from build123d import *

# Parameters (mm, degrees)
SKETCH2_W                      = 127
SKETCH2_H                      = 76.2
BOSS_EXTRUDE2_DEPTH            = 76.2
FILLET1_R                      = 12.7
CHAMFER1_SIZE                  = 10
F_3_4_0_7500_DOWEL_HOLE1_D     = 19.05
F_3_4_0_7500_DOWEL_HOLE1_DEPTH = 76.2
F_3_4_0_7500_DOWEL_HOLE1_TIP   = 5.723197396
SKETCH9_W                      = 38.1
SKETCH9_H                      = 38.1
BOSS_EXTRUDE3_DEPTH            = 76.2
SKETCH10_R                     = 6.355
CUT_EXTRUDE1_DEPTH             = 175.711569487
FILLET3_R                      = 4.76


# Read off the part's stored shape, not the designer's step: 1/4-20 Tapped Hole1
with BuildPart() as part:
    # Sketch2 → Boss-Extrude2 (new body)
    with BuildSketch(Plane(origin=(0, 0, 0), x_dir=(1, 0, 0), z_dir=(0, 1, 0))):
        Rectangle(SKETCH2_W, SKETCH2_H)
    extrude(amount=BOSS_EXTRUDE2_DEPTH)

    # Fillet1
    fillet1_edges = [part.edges().sort_by_distance(p)[0] for p in [
        (-63.5, 76.2, 0),
        (-63.5, 0, 0),
    ]]
    fillet(fillet1_edges, radius=FILLET1_R)

    # Chamfer1
    chamfer1_edges = [part.edges().sort_by_distance(p)[0] for p in [
        (-63.5, 38.1, 38.1),
        (-63.5, 38.1, -38.1),
        (6.35, 0, 38.1),
        (6.35, 76.2, 38.1),
        (-59.780256121, 72.480256121, 38.1),
        (-59.780256121, 3.719743879, 38.1),
        (-59.780256121, 72.480256121, -38.1),
        (-59.780256121, 3.719743879, -38.1),
        (6.35, 0, -38.1),
        (6.35, 76.2, -38.1),
    ]]
    chamfer(chamfer1_edges, length=CHAMFER1_SIZE)

    # 3/4 (0.7500) Dowel Hole1
    with Locations(Plane(origin=(63.5, 0, 0), x_dir=(0, 0, -1), z_dir=(1, 0, 0))):
        with Locations((0, 36.890636669)):
            Hole(F_3_4_0_7500_DOWEL_HOLE1_D / 2, depth=F_3_4_0_7500_DOWEL_HOLE1_DEPTH)
            with Locations((0, 0, -(F_3_4_0_7500_DOWEL_HOLE1_DEPTH + F_3_4_0_7500_DOWEL_HOLE1_TIP / 2))):  # 118° drill point
                Cone(0, F_3_4_0_7500_DOWEL_HOLE1_D / 2, F_3_4_0_7500_DOWEL_HOLE1_TIP, mode=Mode.SUBTRACT)

    # 1/4-20 Tapped Hole1 outline → 1/4-20 Tapped Hole1 (revolve, cut)
    with BuildSketch(Plane(origin=(9.290251981, 0, 0), x_dir=(1, 0, 0), z_dir=(0, 0, 1))):
        Polygon((2.5527, 0), (2.5527, 27.365636669), (2.145213678, 27.610479152), (0, 27.610479152), (0, 0), align=None)
    revolve(axis=Axis((9.290251981, 0, 0), (0, 1, 0)), mode=Mode.SUBTRACT)

    # 1_4-20 Tapped Hole1 2 outline → 1_4-20 Tapped Hole1 2 (revolve, cut)
    with BuildSketch(Plane(origin=(36.474004082, 0, 0), x_dir=(1, 0, 0), z_dir=(0, 0, 1))):
        Polygon((2.5527, 0), (2.5527, 27.365636669), (2.145213678, 27.610479152), (0, 27.610479152), (0, 0), align=None)
    revolve(axis=Axis((36.474004082, 0, 0), (0, 1, 0)), mode=Mode.SUBTRACT)

    # Sketch9 → Boss-Extrude3 (add)
    with BuildSketch(Plane(origin=(0, 76.2, 0), x_dir=(1, 0, 0), z_dir=(0, 1, 0))):
        Rectangle(SKETCH9_W, SKETCH9_H)
    extrude(amount=BOSS_EXTRUDE3_DEPTH)

    # Sketch10 → Cut-Extrude1 (cut, through all)
    with BuildSketch(Plane.XY.offset(19.05)):
        with Locations((0, 98.552)):
            Circle(SKETCH10_R)
        with Locations((0, 130.302)):
            Circle(SKETCH10_R)
    extrude(amount=-CUT_EXTRUDE1_DEPTH, mode=Mode.SUBTRACT)

    # Fillet3
    fillet3_edges = [part.edges().sort_by_distance(p)[0] for p in [
        (19.05, 114.3, 19.05),
        (19.05, 114.3, -19.05),
        (-19.05, 114.3, -19.05),
        (-19.05, 114.3, 19.05),
    ]]
    fillet(fillet3_edges, radius=FILLET3_R)


solid = part.part
Input: part model. Units: mm. Frame: model coordinates. A direction names the side the tool comes from. Coordinates: 2 decimals unless noted, no trailing zeros. Loops run counter-clockwise (first coordinate to the right, second up) from the corner with the lowest first, then second, coordinate; pieces in that order, holes last. Notation, with made-up numbers: (88.5, -28.5) -> (96.5, -28.5) arc R15 cw to (96.5, -16.5) -> close; hole circle Ø4 at (63.25, 35). An arc over 180 degrees is marked (long way). Write item = value, one per line. Start each with the question number.
Item 1: Cut plane B-B, the plane y = 117.5. Return loops of the section in (x, z).
Item 2: Cut plane C-C, the plane x = -31.5. Return loops of the section in (y, z).
Item 3: First-contact query: P1, Ø11.5, axis at x = 0, y = 130.302, coming from the -Z side; P2, Ø23, axis at y = 108.5, z = -6.5, coming from the -X side; P3, Ø8.5, axis at x = 5, y = 111.5, coming from the -Z side; P4, Ø8, axis at x = 36.47, z = 0, coming from the +Y side. Flat tips, straight axial feed; report the tip coordinate or a pass-through.
Item 4: Cut plane A-A, the plane x = 0. Return loops of the section in (y, z) (3 decimals), plus the area to 3 significant figures.
Item 5: Cut plane D-D, the plane x = 16. Return loops of the section in (y, z) (3 decimals).
Item 6: Mould query, pull axis X, two halves, no side actions, for faces 5 (the face through (-4.68, 134.6, 0.27)), 6 (the face through (-17.43, 35.42, -0.76)), 7 (the face through (-56.25, 68.84, -33.17)). Classes: pulls with the +X half, pulls with the -X half, needs draft (parallel to the pull), parting line crosses it, or undercut.
Item 7: Material intervals for line 1 (X direction, y = 16.5, z = 0); line 2 (Y direction, x = 0, z = 5.5); line 3 (Y direction, x = 0, z = -1), sorted ascending.
Item 8: Reachability of faces 1 (the face through (-17.62, 114.83, -17.69)), 2 (the face through (-19.05, 114, 0)), 3 (the face through (0, 114, -19.05)), 4 (the face through (24.9, 27.6, -2.1)) from +Z, -Z, +X, -X, +Y, -Y: full face, straight path, thin tool, end or side. Return the list, or none.
Ans:
q1.outline = (-19.05, -14.29) arc R4.76 ccw to (-14.29, -19.05) -> (14.29, -19.05) arc R4.76 ccw to (19.05, -14.29) -> (19.05, 14.29) arc R4.76 ccw to (14.29, 19.05) -> (-14.29, 19.05) arc R4.76 ccw to (-19.05, 14.29) -> close
q2.outline = (0, -28.1) -> (10, -38.1) -> (66.2, -38.1) -> (76.2, -28.1) -> (76.2, 28.1) -> (66.2, 38.1) -> (10, 38.1) -> (0, 28.1) -> close
q3.P1 = through
q3.P2 = -19.05
q3.P3 = -19.05
q3.P4 = 76.2
q4.outline = (0, -28.1) -> (10, -38.1) -> (66.2, -38.1) -> (76.2, -28.1) -> (76.2, -19.05) -> (92.197, -19.05) -> (92.197, 19.05) -> (76.2, 19.05) -> (76.2, 28.1) -> (66.2, 38.1) -> (10, 38.1) -> (0, 28.1) -> close; (104.907, -19.05) -> (123.947, -19.05) -> (123.947, 19.05) -> (104.907, 19.05) -> close; (136.657, -19.05) -> (152.4, -19.05) -> (152.4, 19.05) -> (136.657, 19.05) -> close; hole circle Ø19.05 at (36.891, 0)
q4.area = 7,260 mm²
q5.outline = (0, -28.1) -> (10, -38.1) -> (66.2, -38.1) -> (76.2, -28.1) -> (76.2, -18.732) -> (152.4, -18.732) -> (152.4, 18.732) -> (76.2, 18.732) -> (76.2, 28.1) -> (66.2, 38.1) -> (10, 38.1) -> (0, 28.1) -> close; hole circle Ø19.05 at (36.891, 0)
q6.face_5 = undercut
q6.face_6 = pulls with the +X half
q6.face_7 = pulls with the -X half
q7.line_1 = -63.5 to 6.74, 11.84 to 33.92, 39.03 to 63.5
q7.line_2 = 0 to 29.11, 44.67 to 92.2, 104.91 to 123.95, 136.66 to 152.4
q7.line_3 = 0 to 27.42, 46.36 to 92.2, 104.91 to 123.95, 136.66 to 152.4
q8.face_1 = -Z, -X, +Y
q8.face_2 = +Z, -Z, -X, +Y
q8.face_3 = -Z, +X, -X, +Y
q8.face_4 = +X
